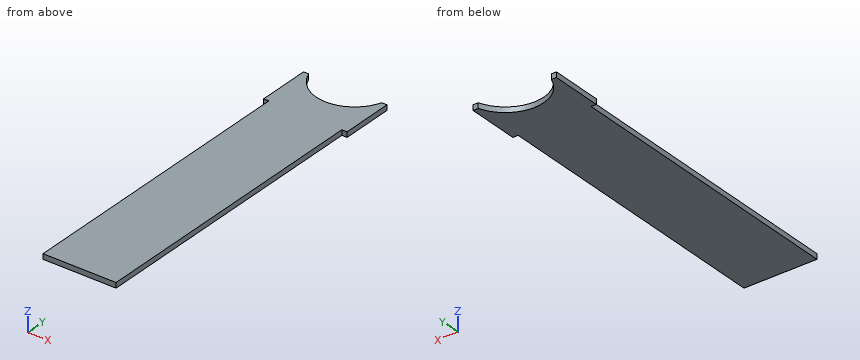
from build123d import *

# Parameters (mm, degrees)
SKETCH2_W           = 1.5875
SKETCH2_H           = 15.875
BOSS_EXTRUDE1_DEPTH = 1.5875


with BuildPart() as part:
    # Sketch2 → Boss-Extrude1 (new body)
    with BuildSketch(Plane.XY):
        with BuildLine():
            ThreePointArc((11.1125, 0), (0, -7.9375), (-11.1125, 0))
            Line((-11.1125, 0), (-11.1125, -15.875))
            Line((-11.1125, -15.875), (-11.1125, -105.804584263))
            Line((-11.1125, -105.804584263), (11.1125, -105.804584263))
            Line((11.1125, -105.804584263), (11.1125, -15.875))
            Line((11.1125, -15.875), (11.1125, 0))
        make_face()
        with Locations((-11.90625, -7.9375)):
            Rectangle(SKETCH2_W, SKETCH2_H)
        with Locations((11.90625, -7.9375)):
            Rectangle(SKETCH2_W, SKETCH2_H)
    extrude(amount=BOSS_EXTRUDE1_DEPTH)


solid = part.part
Verification items for the finished model (mm, model axes). Give positions to 0.01 mm unless a question says otherwise; leave off trailing zeros. Write each loop counter-clockwise with the first axis right and the second up, starting at its lowest first coordinate (ties: lowest second). Pieces come first, ordered by that corner, then holes. Notation, with made-up numbers: M -22,88.25 L -3,88.25 A22 ccw -3,126.25 Z; hole C -32.75,-26.75 d2. An arc over 180 degrees is marked long. Put each result on its own line as item: value. Start each with the question number.
1. Section check C-C (x = -10). Record the cut outline in (y, z).
2. Section check B-B (y = -66.5). Record the cut outline in (x, z).
3. Go/stop test with flat-tipped pins: pin 1 Ø0.8 at (x, z) = (12, 0.5) entering from -Y (3 decimals); pin 2 Ø0.8 at (y, z) = (-57, 0.5) entering from -X. Record where each tip stops, or that it passes through.
4. Scan lines: line 1 along X through (y, z) = (-59.5, 0.85); line 2 along Y through (x, z) = (0, 0.25); line 3 along Y through (x, z) = (11.5, 0.85) (3 decimals). Record each from-to range of solid material in increasing order. Write a range as [from, to].
5. Section check A-A (z = 0.7). Record the cut outline in (x, y) (1 decimal), and give its area (3 significant figures).
Answer list:
1. outline: M -105.8,0 L -2.35,0 L -2.35,1.59 L -105.8,1.59 Z
2. outline: M -11.11,0 L 11.11,0 L 11.11,1.59 L -11.11,1.59 Z
3. pin 1: y = -15.875
3. pin 2: x = -11.11
4. line 1: [-11.11, 11.11]
4. line 2: [-105.8, -7.94]
4. line 3: [-15.875, 0]
5. outline: M -12.7,-15.9 L -11.1,-15.9 L -11.1,-105.8 L 11.1,-105.8 L 11.1,-15.9 L 12.7,-15.9 L 12.7,0 L 11.1,0 A11.7 cw -11.1,0 L -12.7,0 Z
5. area: 2,270 mm2
